```python
from build123d import *

# Parameters (mm, degrees)
F0_W      = 844.55
F0_H      = 85.725
F1_DEPTH  = 25.4
F2_W      = 12.7
F2_H      = 50.8
F3_DEPTH  = 25.401
F4_W      = 12.7
F4_H      = 6.35
F5_DEPTH  = 85.726
F6_R      = 4.564063
F7_DEPTH  = 50.8
F8_R      = 12.7
F9_DEPTH  = 19.05
F10_W     = 812.8
F10_H     = 25.4
F11_DEPTH = 12.7


with BuildPart() as f1:
    # F0 (on Front) → F1 (new body)
    with BuildSketch(Plane.XZ):
        with Locations((422.275, 42.8625)):
            Rectangle(F0_W, F0_H)
    extrude(amount=F1_DEPTH)

    # F2 (on face) → F3 (cut, through all)
    with BuildSketch(Plane.XZ.offset(25.4)):
        with Locations((6.35, 60.325)):
            Rectangle(F2_W, F2_H)
        with Locations((838.2, 60.325)):
            Rectangle(F2_W, F2_H)
    extrude(amount=-F3_DEPTH, mode=Mode.SUBTRACT)

    # F4 (on face) → F5 (cut, through all)
    with BuildSketch(Plane(origin=(0, 0, 0), x_dir=(1, 0, 0), z_dir=(0, 0, -1))):
        with Locations((838.2, 22.225)):
            Rectangle(F4_W, F4_H)
        with Locations((838.2, 3.175)):
            Rectangle(F4_W, F4_H)
        with Locations((6.35, 22.225)):
            Rectangle(F4_W, F4_H)
        with Locations((6.35, 3.175)):
            Rectangle(F4_W, F4_H)
    extrude(amount=-F5_DEPTH, mode=Mode.SUBTRACT)

    # F6 (on face) → F7 (cut)
    with BuildSketch(Plane(origin=(12.7, 0, 0), x_dir=(0, -1, 0), z_dir=(-1, 0, 0))):
        with Locations((12.7, 60.325)):
            Circle(F6_R)
    extrude(amount=-F7_DEPTH, mode=Mode.SUBTRACT)

    # F8 (on face) → F9 (cut)
    with BuildSketch(Plane(origin=(0, 0, 0), x_dir=(-1, 0, 0), z_dir=(0, 1, 0))):
        with Locations((-66.675, 60.325)):
            Circle(F8_R)
        with Locations((-777.875, 60.325)):
            Circle(F8_R)
    extrude(amount=-F9_DEPTH, mode=Mode.SUBTRACT)

    # F10 (on face) → F11 (join)
    with BuildSketch(Plane(origin=(0, 0, 0), x_dir=(-1, 0, 0), z_dir=(0, 1, 0))):
        with Locations((-422.275, 28.575)):
            Rectangle(F10_W, F10_H)
    extrude(amount=F11_DEPTH)


solid = f1.part
```
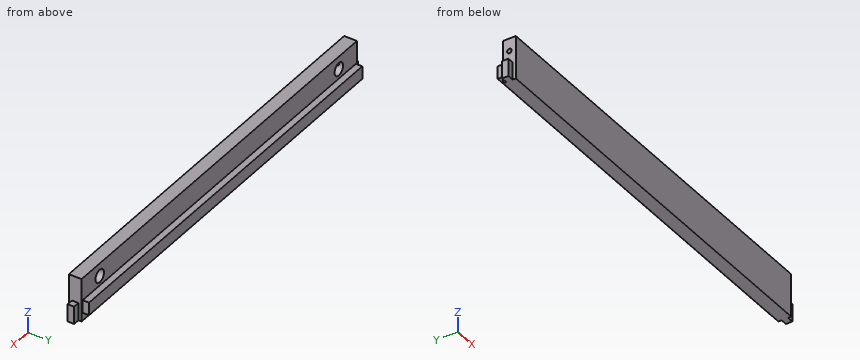
Part model, mm, in its own coordinate system. Give positions to 0.01 mm unless a question says otherwise; leave off trailing zeros. Write each loop counter-clockwise with the first axis right and the second up, starting at its lowest first coordinate (ties: lowest second). Pieces come first, ordered by that corner, then holes. Notation, with made-up numbers: (-10.5, 18) -> (39.5, 18) arc R18 cw to (39.5, 24) -> close; hole circle Ø4 at (28.25, 1). An arc over 180 degrees is marked (long way). Put each result on its own line as item: value. Start each with the question number.
Item 1: Pin check, flat tips, straight feed: pin 1 Ø8 at (y, z) = (0, 63.5) entering from -X; pin 2 Ø12.5 at (x, z) = (63.5, 61) entering from +Y; pin 3 Ø6.5 at (x, y) = (837, -12.5) entering from +Z (3 decimals). Stop position of each tip, or through.
Item 2: Wall check: L1, parallel to X at y = -0.5, z = 61.5; L2, parallel to Y at x = 516, z = 13.5; L3, parallel to Z at x = 537, y = 1 (3 decimals). Give the ranges that are in metal, low to high. Write a range as [from, to].
Item 3: Cut at A-A (x = 239). List the corners of the cut face in (y, z) (3 decimals).
Answer list:
1. pin 1: stops at x = 12.7
1. pin 2: stops at y = -19.05
1. pin 3: stops at z = 34.925
2. L1: x = [12.7, 54.03], [79.32, 765.23], [790.52, 831.85]
2. L2: y = [-25.4, 0]
2. L3: z = [15.875, 41.275]
3. outline: (-25.4, 0) -> (0, 0) -> (0, 15.875) -> (12.7, 15.875) -> (12.7, 41.275) -> (0, 41.275) -> (0, 85.725) -> (-25.4, 85.725) -> close
